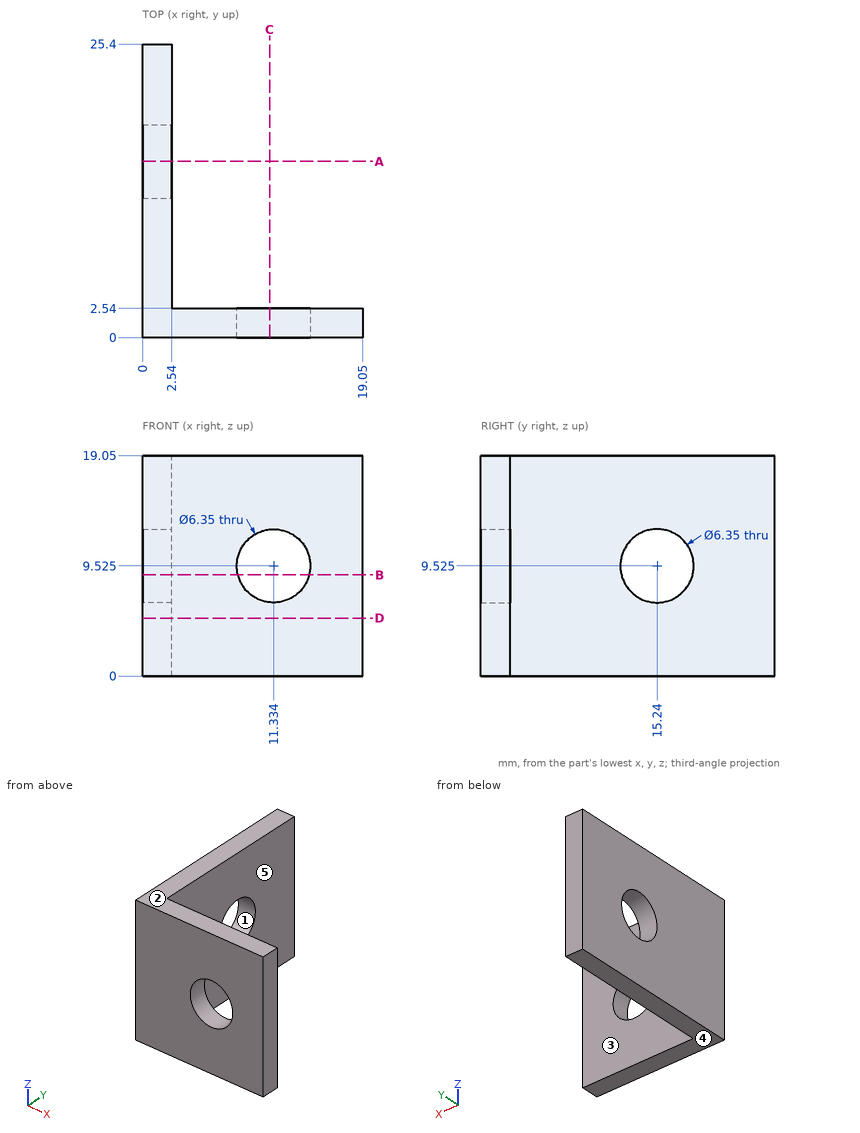
Verification items for this drawing (mm, ordinates from the low corner). A direction names the side the tool comes from. Coordinates: 2 decimals unless noted, no trailing zeros. Write each loop counter-clockwise with the first axis right and the second up, starting at its lowest first coordinate (ties: lowest second). Pieces come first, ordered by that corner, then holes. Notation, with made-up numbers: (22.5, -8) -> (51.5, -8) arc R22 ccw to (51.5, -1) -> close; hole circle Ø5 at (12, 26.25). An arc over 180 degrees is marked (long way). One line per item, written item: value. Start each with the question number.
Q1. Mould release check, pull along Z, two halves, no side actions. Record for the marked faces 1, 2 and 3: pulls with the +Z half, pulls with the -Z half, needs draft (parallel to the pull), parting line crosses it, or undercut.
Q2. Access from +Z, -Z, +X, -X, +Y, -Y to the whole of each face (thin tool, end or side, straight path). Record for the marked faces 4 and 5.
Q3. Cross-section at B-B on z = 8.75. State how many separate pieces and enclosed holes the cut face has.
Q4. Thickness scan on L1, parallel to Y at x = 11.25, z = 14; L2, parallel to X at y = 1.5, z = 11.5. Record the ranges inside material, lowest first. Write a range as from..to.
Q5. Cross-section at A-A on y = 15.24. Enter the section's corners in (x, z).
Q6. Cross-section at C-C on x = 11. Enter the section's corners in (y, z).
Q7. Go/stop test with flat-tipped pins: P1, Ø3, axis at y = 22.5, z = 9, coming from the -X side; P2, Ø3, axis at x = 16.5, z = 8.5, coming from the +Y side; P3, Ø3, axis at y = 21.5, z = 6, coming from the +X side. Record where each tip stops, or that it passes through.
Q8. Cross-section at D-D on z = 5. Enter the section's corners in (x, y), and give its area (3 significant figures).
Checked values:
1. face 1: undercut
1. face 2: pulls with the +Z half
1. face 3: needs draft
2. face 4: -Z, +X, -X, +Y, -Y
2. face 5: +Z, -Z, +X, +Y
3. separate pieces: 3
3. enclosed holes: 0
4. L1: y = 0..2.54
4. L2: x = 0..8.85, 13.82..19.05
5. outline: (0, 0) -> (2.54, 0) -> (2.54, 6.35) -> (0, 6.35) -> close; (0, 12.7) -> (2.54, 12.7) -> (2.54, 19.05) -> (0, 19.05) -> close
6. outline: (0, 0) -> (2.54, 0) -> (2.54, 6.37) -> (0, 6.37) -> close; (0, 12.68) -> (2.54, 12.68) -> (2.54, 19.05) -> (0, 19.05) -> close
7. P1: stops at x = 0
7. P2: stops at y = 2.54
7. P3: stops at x = 2.54
8. outline: (0, 0) -> (19.05, 0) -> (19.05, 2.54) -> (2.54, 2.54) -> (2.54, 25.4) -> (0, 25.4) -> close
8. area: 106 mm²
